```python
from build123d import *

# Parameters (mm, degrees)
SKETCH1_W           = 300
SKETCH1_H           = 120
SKETCH1_R           = 13.75
SKETCH1_W_2         = 35
SKETCH1_H_2         = 6
SKETCH1_W_3         = 40
SKETCH1_H_3         = 40
SKETCH1_H_4         = 2
BOSS_EXTRUDE1_DEPTH = 5
SKETCH3_R           = 15.75
SKETCH3_R_2         = 13.75
SKETCH3_W           = 44
SKETCH3_H           = 44
SKETCH3_W_2         = 40
SKETCH3_H_2         = 40
BOSS_EXTRUDE5_DEPTH = 10


with BuildPart() as part:
    # Sketch1 → Boss-Extrude1 (new body)
    with BuildSketch(Plane(origin=(0, 0, 0), x_dir=(1, 0, 0), z_dir=(0, 1, 0))):
        Rectangle(SKETCH1_W, SKETCH1_H)
        with Locations(Location((24.074387053, -14.407309066, 0), (0, 0, 270))):
            Circle(SKETCH1_R, mode=Mode.SUBTRACT)
        with Locations((-87.5, 52)):
            Rectangle(SKETCH1_W_2, SKETCH1_H_2, mode=Mode.SUBTRACT)
        with Locations((87.5, 52)):
            Rectangle(SKETCH1_W_2, SKETCH1_H_2, mode=Mode.SUBTRACT)
        with Locations((-110, -25)):
            Rectangle(SKETCH1_W_3, SKETCH1_H_3, mode=Mode.SUBTRACT)
        with Locations((0, 23.756786453)):
            Rectangle(SKETCH1_W_3, SKETCH1_H_4, mode=Mode.SUBTRACT)
    extrude(amount=BOSS_EXTRUDE1_DEPTH)

    # Sketch3 → Boss-Extrude5 (add)
    # profile 1 of 2: a face of its own
    with BuildSketch(Plane(origin=(0, 5, 0), x_dir=(1, 0, 0), z_dir=(0, 1, 0))):
        with Locations(Location((24.074387053, -14.407309066, 0), (0, 0, 90))):
            Circle(SKETCH3_R)
        with Locations(Location((24.074387053, -14.407309066, 0), (0, 0, 270))):
            Circle(SKETCH3_R_2, mode=Mode.SUBTRACT)
    # profile 2 of 2: a face of its own
    with BuildSketch(Plane(origin=(0, 5, 0), x_dir=(1, 0, 0), z_dir=(0, 1, 0))):
        with Locations((-110, -25)):
            Rectangle(SKETCH3_W, SKETCH3_H)
        with Locations((-110, -25)):
            Rectangle(SKETCH3_W_2, SKETCH3_H_2, mode=Mode.SUBTRACT)
    extrude(amount=BOSS_EXTRUDE5_DEPTH)


solid = part.part
```
Geometry check sheet. Reference: the model listing, model coordinates, mm. A direction names the side the tool comes from. Coordinates: 2 decimals unless noted, no trailing zeros. Write each loop counter-clockwise with the first axis right and the second up, starting at its lowest first coordinate (ties: lowest second). Pieces come first, ordered by that corner, then holes. Notation, with made-up numbers: M 19,-1.75 L 37,-1.75 A14 ccw 37,20.25 Z; hole C 44,-1 d4. An arc over 180 degrees is marked long. Use one line per item in the form item = value. Start each with the question number.
1) Set-up check for faces 1 (the flat face through (-112, 15, 46)), 2 (the flat face through (-110, 10, 47)), 3 (the cylindrical face through (38.047, 9.93, 7.14)), 4 (the flat face through (0, 2, -22.757)), 5 (the flat face through (-2, 0, -1)): record each of +Z, -Z, +X, -X, +Y, -Y from which the full face is reachable in a straight line by a thin tool's end or side.
2) Section check A-A on x = 2. Enter the section's corners in (y, z), and give its area (3 significant figures).
3) Section check B-B on z = 41. Enter the section's corners in (x, y).
4) Section check D-D on x = 81. Enter the section's corners in (y, z).
5) Go/stop test with flat-tipped pins: pin 1 Ø25 at (x, z) = (24.07, 14.41) entering from -Y; pin 2 Ø8 at (x, y) = (-109.5, 12) entering from -Z; pin 3 Ø7.5 at (x, y) = (-104, 9) entering from +Z; pin 4 Ø5 at (y, z) = (13, 24.5) entering from -X. Record where each tip stops, or that it passes through.
6) Section check C-C on y = 9.25. Enter the section's corners in (x, z), and give its area (3 significant figures).
7) Thickness scan on probe 1 along Z at (x, y) = (-91.5, 4.5); probe 2 along Z at (x, y) = (0, 4.5); probe 3 along Z at (x, y) = (-125.5, 2). Record the ranges inside material, lowest first. Write a range as from..to.
8) Release check for a two-part mould opening along Z. For faces 6 (the flat face through (-110, 10, 3)), 7 (the flat face through (87, 2, -55)), 8 (the flat face through (-132, 10, 25)) record: pulls with the +Z half, pulls with the -Z half, needs draft (parallel to the pull), parting line crosses it, or undercut.
Responses:
q1.face_1 = +Z, -Z, +X, -X, +Y
q1.face_2 = +Z, +X, -X, +Y
q1.face_3 = +Y
q1.face_4 = +Y, -Y
q1.face_5 = +Z, -Z, +X, -X, -Y
q2.outline = M 0,-60 L 5,-60 L 5,-24.76 L 0,-24.76 Z; M 0,-22.76 L 5,-22.76 L 5,60 L 0,60 Z
q2.area = 590 mm2
q3.outline = M -150,0 L -130,0 L -130,15 L -132,15 L -132,5 L -150,5 Z; M -90,0 L 150,0 L 150,5 L -88,5 L -88,15 L -90,15 Z
q4.outline = M 0,-60 L 5,-60 L 5,-55 L 0,-55 Z; M 0,-49 L 5,-49 L 5,60 L 0,60 Z
q5.pin_1 = through
q5.pin_2 = 3
q5.pin_3 = 47
q5.pin_4 = -132
q6.outline = M -132,3 L -88,3 L -88,47 L -132,47 Z; C 24.07,14.41 d31.5; hole M -130,5 L -90,5 L -90,45 L -130,45 Z; hole C 24.07,14.41 d27.5
q6.area = 521 mm2
q7.probe_1 = -60..-55, -49..5, 45..60
q7.probe_2 = -60..-24.76, -22.76..60
q7.probe_3 = -60..5, 45..60
q8.face_6 = pulls with the -Z half
q8.face_7 = undercut
q8.face_8 = needs draft
